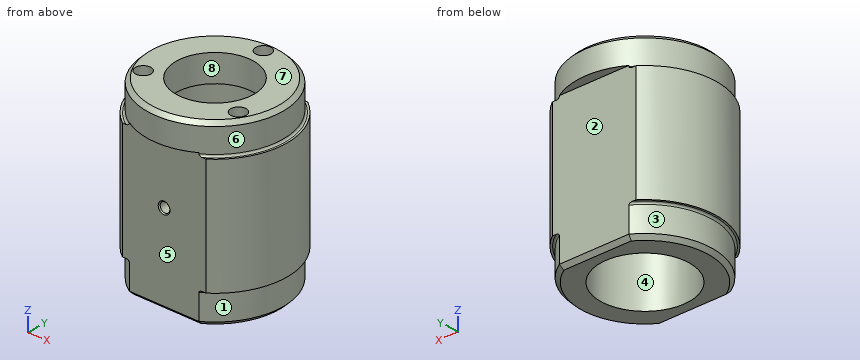
from build123d import *

# Parameters (mm, degrees)
BOSS_EXTRUDE1_DEPTH         = 22.75
BOSS_EXTRUDE1_DEPTH_BACK    = 23
BOSS_EXTRUDE2_DEPTH         = 15
BOSS_EXTRUDE2_DEPTH_BACK    = 15
BOSS_EXTRUDE3_START         = -7
SKETCH5_R                   = 11.5
SKETCH5_R_2                 = 10.000000000000004
BOSS_EXTRUDE3_DEPTH         = 7
SKETCH6_R                   = 2
SKETCH6_R_2                 = 2.0000000000012577
SKETCH6_R_3                 = 2.0000000000018354
CUT_EXTRUDE1_DEPTH          = 5
M3_TAPPED_HOLE1_D           = 2.5
M3_TAPPED_HOLE1_DEPTH       = 7.5
M3_TAPPED_HOLE1_CSINK_D     = 3.05
M3_TAPPED_HOLE1_CSINK_ANGLE = 90
M3_TAPPED_HOLE1_TIP         = 0.7510757737844503
FILLET2_R                   = 0.5
CHAMFER1_SIZE               = 1
CHAMFER2_SIZE               = 1


with BuildPart() as part:
    # Sketch1 → Boss-Extrude1 (new, two sides: drawn at the far end of the back side and taken through both)
    with BuildSketch(Plane.XY.offset(-BOSS_EXTRUDE1_DEPTH_BACK)):
        with BuildLine():
            Line((9.013878188660517, 15), (0, 15))
            Line((0, 15), (0, 11.5))
            ThreePointArc((-1.9847e-13, 11.5), (8.131727983645227, 8.131727983645368), (11.5, 0))
            ThreePointArc((11.5, -2.82e-15), (8.131727983645224, -8.13172798364537), (-2.0639e-13, -11.5))
            Line((0, -11.5), (0, -15))
            Line((0, -14.999999999999998), (9.013878188660513, -14.999999999999996))
            ThreePointArc((9.013878188660447, -14.999999999999721), (15.231429156542696, -8.617050878880846), (17.500000000000004, -4.29e-15))
            ThreePointArc((17.500000000000004, 0), (15.231429156542696, 8.617050878880846), (9.013878188660442, 14.999999999999723))
        make_face()
        with BuildLine():
            Line((0, 11.5), (0, 15))
            Line((0, 15), (-9.013878188659975, 15))
            ThreePointArc((-9.013878188659975, 15.000000000000002), (-17.500000000000004, 1.769e-14), (-9.01387818866, -14.99999999999999))
            Line((-9.013878188659985, -15), (0, -14.999999999999998))
            Line((0, -15), (0, -11.5))
            ThreePointArc((-2.0639e-13, -11.5), (-11.5, 1.41e-15), (-1.9592e-13, 11.5))
        make_face()
    extrude(amount=BOSS_EXTRUDE1_DEPTH + BOSS_EXTRUDE1_DEPTH_BACK)

    # Sketch1_23 → Boss-Extrude2 (add, two sides: drawn at the far end of the back side and taken through both)
    with BuildSketch(Plane.XY.offset(-BOSS_EXTRUDE2_DEPTH_BACK)):
        with BuildLine():
            Line((-9.013878188659975, 15), (-10.828203913853855, 15))
            ThreePointArc((-10.828203913853855, 15.000000000000004), (-18.5, -5.95e-15), (-10.828203913853852, -15.000000000000005))
            Line((-10.828203913853855, -15), (-9.013878188659985, -15))
            ThreePointArc((-9.01387818866, -14.99999999999999), (-17.500000000000004, 1.769e-14), (-9.013878188659975, 15.000000000000002))
        make_face()
        with BuildLine():
            ThreePointArc((18.5, 0), (16.470758519362374, 8.424020049646833), (10.828203913853855, 15))
            Line((10.828203913853855, 15), (9.013878188660517, 15))
            ThreePointArc((9.013878188660442, 14.999999999999723), (15.231429156542696, 8.617050878880846), (17.500000000000004, 0))
            ThreePointArc((17.500000000000004, -4.29e-15), (15.231429156542696, -8.617050878880846), (9.013878188660447, -14.999999999999721))
            Line((9.013878188660513, -14.999999999999996), (10.828203913853855, -14.999999999999996))
            ThreePointArc((10.828203913853848, -15.000000000000009), (16.47075851936237, -8.42402004964684), (18.5, -4.53e-15))
        make_face()
    extrude(amount=BOSS_EXTRUDE2_DEPTH + BOSS_EXTRUDE2_DEPTH_BACK)

    # Sketch5 → Boss-Extrude3 (add)
    # profile 1 of 3: a face of its own
    with BuildSketch(Plane.XY.offset(22.75).offset(BOSS_EXTRUDE3_START)):
        with BuildLine():
            ThreePointArc((9.01387818866041, 14.999999999999744), (2.5313e-13, 17.500000000000004), (-9.013878188659977, 15.000000000000004))
            Line((-9.013878188659977, 15.000000000000002), (9.013878188660446, 14.999999999999803))
        make_face()
    # profile 2 of 3: a face of its own
    with BuildSketch(Plane.XY.offset(22.75).offset(BOSS_EXTRUDE3_START)):
        Circle(SKETCH5_R)
        Circle(SKETCH5_R_2, mode=Mode.SUBTRACT)
    # profile 3 of 3: a face of its own
    with BuildSketch(Plane.XY.offset(22.75).offset(BOSS_EXTRUDE3_START)):
        with BuildLine():
            ThreePointArc((-9.013878188659994, -14.999999999999993), (2.4336e-13, -17.500000000000004), (9.013878188660414, -14.99999999999974))
            Line((9.013878188660449, -14.999999999999806), (-9.013878188659994, -14.999999999999995))
        make_face()
    extrude(amount=BOSS_EXTRUDE3_DEPTH)

    # Sketch6 → Cut-Extrude1 (cut)
    with BuildSketch(Plane.XY.offset(22.75)):
        with Locations((0, 14.25)):
            Circle(SKETCH6_R)
        with Locations((12.340862003929768, -7.124999999999125)):
            Circle(SKETCH6_R_2)
        with Locations((-12.340862003926736, -7.12500000000088)):
            Circle(SKETCH6_R_3)
    extrude(amount=-CUT_EXTRUDE1_DEPTH, mode=Mode.SUBTRACT)

    # M3 Tapped Hole1
    with Locations(Plane(origin=(2.4e-15, -14.999999999999998, 0), x_dir=(-1, -1.6e-16, 0), z_dir=(1.6e-16, -1, 0))):
        with Locations((0, 0)):
            CounterSinkHole(M3_TAPPED_HOLE1_D / 2, M3_TAPPED_HOLE1_CSINK_D / 2, depth=M3_TAPPED_HOLE1_DEPTH, counter_sink_angle=M3_TAPPED_HOLE1_CSINK_ANGLE)
            with Locations((0, 0, -(M3_TAPPED_HOLE1_DEPTH + M3_TAPPED_HOLE1_TIP / 2))):  # 118° drill point
                Cone(0, M3_TAPPED_HOLE1_D / 2, M3_TAPPED_HOLE1_TIP, mode=Mode.SUBTRACT)

    # Fillet2
    fillet2_edges = [part.edges().sort_by_distance(p)[0] for p in [
        (17.500000000000004, 5.77e-15, 15),
        (17.500000000000007, -3.55e-15, -15),
        (-17.5, 1.821e-14, 15),
        (-17.5, 1.821e-14, -15),
    ]]
    fillet(fillet2_edges, radius=FILLET2_R)

    # Chamfer1
    chamfer1_edges = [part.edges().sort_by_distance(p)[0] for p in [
        (-17.500000000000007, 1.066e-14, -23),
        (9.01387818866, 14.99999999999999, 22.75),
        (17.500000000000004, 5.77e-15, -23),
    ]]
    chamfer(chamfer1_edges, length=CHAMFER1_SIZE)

    # Chamfer2
    chamfer2_edges = [part.edges().sort_by_distance(p)[0] for p in [
        (7.11e-15, -14.999999999999927, -23),
        (1.421e-14, 14.999999999999932, -23),
    ]]
    chamfer(chamfer2_edges, length=CHAMFER2_SIZE)


solid = part.part
Source: CAD feature listing. Evaluate the final solid. Frame: model axes, mm. Face numbers are marked on the shaded views. A direction names the side the tool comes from. Round coordinates to 2 decimals unless told otherwise and drop trailing zeros. Loops run counter-clockwise (first coordinate to the right, second up) from the corner with the lowest first, then second, coordinate; pieces in that order, holes last.
Q1. Section D-D, the plane z = 17. Return loops of the section in (x, y).
Q2. Section B-B, the plane z = 0. Return loops of the section in (x, y) (3 decimals).
Q3. Section C-C, the plane z = 8. Return loops of the section in (x, y), plus the area to 3 significant figures.
Q4. First-contact query: P1, Ø1.3, axis at x = -3, y = 16.5, coming from the -Z side; P2, Ø17.5, axis at x = -3, z = 0.5, coming from the +Y side; P3, Ø1, axis at y = 5, z = 4.5, coming from the +X side; P4, Ø2, axis at x = -13, y = -8, coming from the +Z side. Flat tips, straight axial feed; report the tip coordinate or a pass-through.
Q5. Ray query, line 1 (Y direction, x = 0, z = 20.95); line 2 (Z direction, x = 0, y = -12.75); line 3 (Z direction, x = 12, y = -8). Return the intervals inside material, ascending.
Q6. Access query for the marked faces 1, 2, 3, 4 and 5. Directions: +Z, -Z, +X, -X, +Y, -Y. A direction counts if a zero-diameter tool reaches every point of the face in a straight line with its end or side. Return the directions, or none.
Q7. Section A-A, the plane x = 0. State how many separate pieces and enclosed holes the cut face has, plus the area to 3 significant figures.
Q8. Mould query, pull axis X, two halves, no side actions, for the marked faces 6, 7 and 8. Classes: pulls with the +X half, pulls with the -X half, needs draft (parallel to the pull), parting line crosses it, or undercut.
Solutions:
1. outline: circle Ø35 at (0, 0); hole circle Ø20 at (0, 0)
2. outline: (-10.828, -15) - (-1.525, -15) - (-1.25, -14.725) - (-1.25, -11.432) arc R11.5 cw (long way) to (1.25, -11.432) - (1.25, -14.725) - (1.525, -15) - (10.828, -15) arc R18.5 ccw to (10.828, 15) - (-10.828, 15) arc R18.5 ccw to start
3. outline: (-10.83, -15) - (10.83, -15) arc R18.5 ccw to (10.83, 15) - (-10.83, 15) arc R18.5 ccw to start; hole circle Ø23 at (0, 0)
3. area: 557 mm2
4. P1: stops at z = 15.75
4. P2: stops at y = 15
4. P3: stops at x = 17.94
4. P4: stops at z = 22.75
5. line 1: y = -17.5 to -10, 10 to 12.25, 16.25 to 17.5
5. line 2: z = -23 to -1.25, 1.25 to 22.75
5. line 3: z = -23 to 17.75
6. face 1: -Z, +X
6. face 2: -Z, +X, -X, +Y
6. face 3: -Z, -X
6. face 4: -Z
6. face 5: -Z, +X, -X, -Y
7. separate pieces: 3
7. enclosed holes: 0
7. area: 345 mm2
8. face 6: parting line crosses it
8. face 7: needs draft
8. face 8: undercut
